Print and shaded views of the part. All mm, measured from the part's lowest x, y and z. Coordinates: 2 decimals unless noted, no trailing zeros. Order: outer loops, then holes, each group sorted by start corner. A loop starts at its lowest first (then second) coordinate and runs counter-clockwise, first axis right, second up.
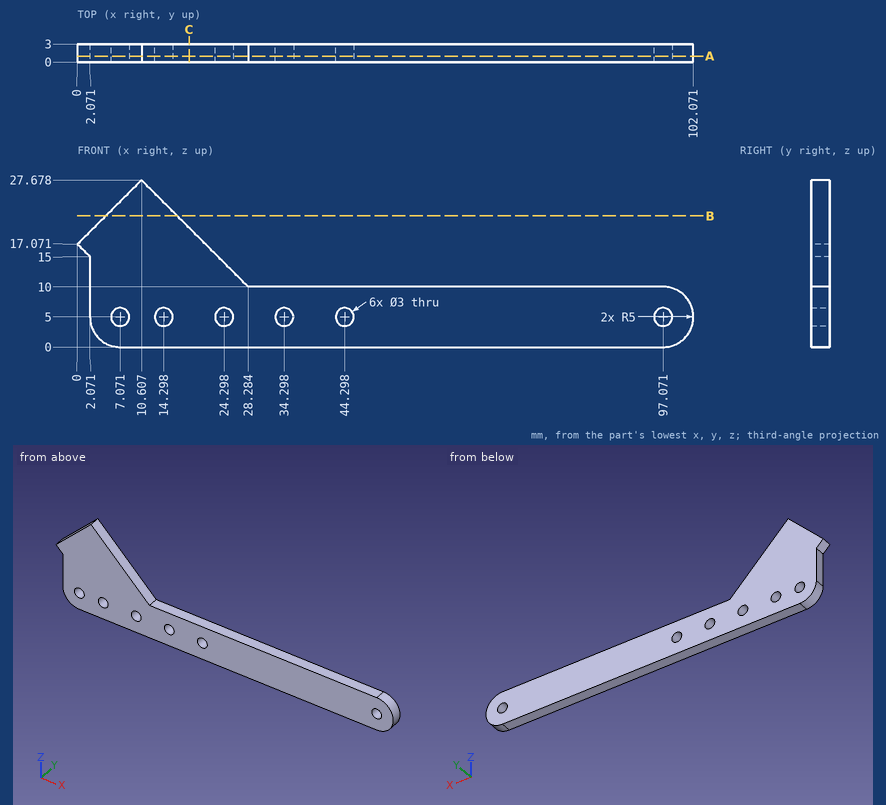
Q1. Drop flat-ended pins along their axis: P1, Ø1.8, axis at x = 97.07, z = 5, coming from the -Y side; P2, Ø1.5, axis at y = 1.5, z = 22, coming from the +X side (1 decimal); P3, Ø1.5, axis at y = 1.5, z = 6, coming from the -X side; P4, Ø1.5, axis at x = 47, y = 1, coming from the +Z side. Give the stop position or say it passes through.
Established:
P1: passes through
P2: stops at x = 17
P3: stops at x = 2.07
P4: stops at z = 10
Q2. Cut at C-C, the plane x = 18.5. List the corners of the cut face in (y, z) (1 decimal).
Established:
outline: (0, 0) - (3, 0) - (3, 19.8) - (0, 19.8) - close
Q3. Cut at A-A, the plane y = 1. List the corners of the cut face in (x, z) (1 decimal), plus the area to 3 significant figures.
Established:
outline: (0, 17.1) - (2.1, 15) - (2.1, 5) arc R5 ccw to (7.1, 0) - (97.1, 0) arc R5 ccw to (97.1, 10) - (28.3, 10) - (10.6, 27.7) - close; hole circle Ø3 at (7.1, 5); hole circle Ø3 at (14.3, 5); hole circle Ø3 at (24.3, 5); hole circle Ø3 at (34.3, 5); hole circle Ø3 at (44.3, 5); hole circle Ø3 at (97.1, 5)
area: 1,220 mm2
Q4. Cut at B-B, the plane z = 21.75. List the corners of the cut face in (x, y) (1 decimal).
Established:
outline: (4.7, 0) - (16.5, 0) - (16.5, 3) - (4.7, 3) - close
Q5. Probe line 1 (Z direction, x = 68.5, y = 2.1); line 2 (Z direction, x = 33.5, y = 0.8); line 3 (Z direction, x = 33, y = 1.35). List the from-to ranges inside material, lowest first.
Established:
line 1: z = 0 to 10
line 2: z = 0 to 3.73, 6.27 to 10
line 3: z = 0 to 4.25, 5.75 to 10
